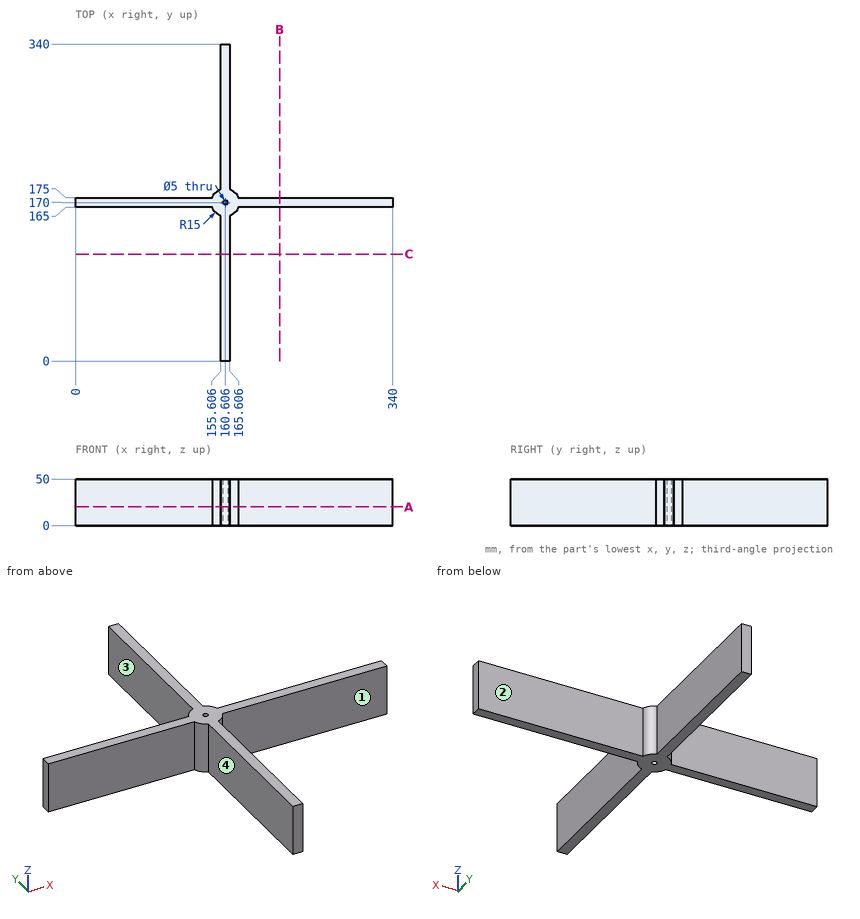
Verification items for this drawing (mm, ordinates from the low corner). A direction names the side the tool comes from. Give positions to 0.01 mm unless a question says otherwise; leave off trailing zeros. Loops run counter-clockwise (first coordinate to the right, second up) from the corner with the lowest first, then second, coordinate; pieces in that order, holes last. Notation, with made-up numbers: M 21.5,-31.5 L 62.5,-31.5 A22 ccw 62.5,-4.5 Z; hole C -11.5,31.25 d2. An arc over 180 degrees is marked long. Answer in a Markdown table with one row per item.
1) Thickness scan on line 1 (X direction, y = 170, z = 24); line 2 (X direction, y = 113, z = 5); line 3 (Y direction, x = 265.5, z = 2). Record the ranges inside material, lowest first.
Solutions:
| item | result |
|---|---|
| line 1 | x = 0 to 158.11, 163.11 to 340 |
| line 2 | x = 155.61 to 165.61 |
| line 3 | y = 165 to 175 |
2) Cross-section at A-A (z = 20). Enter the section's corners in (x, y), plus the area to 3 significant figures.
Solutions:
| item | result |
|---|---|
| outline | M 0,165 L 146.46,165 A15 ccw 155.61,155.86 L 155.61,0 L 165.61,0 L 165.61,155.86 A15 ccw 174.75,165 L 340,165 L 340,175 L 174.75,175 A15 ccw 165.61,184.14 L 165.61,340 L 155.61,340 L 155.61,184.14 A15 ccw 146.46,175 L 0,175 Z; hole C 160.61,170 d5 |
| area | 6,900 mm^2 |
3) Cross-section at C-C (y = 114.5). Enter the section's corners in (x, z).
Solutions:
| item | result |
|---|---|
| outline | M 155.61,0 L 165.61,0 L 165.61,50 L 155.61,50 Z |
4) Tool access check on the marked faces 1, 2, 3 and 4. Record the directions out of +Z, -Z, +X, -X, +Y, -Y that give a thin tool (end or side, any length) a straight path to the whole face; none if there is none.
Solutions:
| item | result |
|---|---|
| face 1 | +Z, -Z, +X, -Y |
| face 2 | +Z, -Z, +X, +Y |
| face 3 | +Z, -Z, -X, +Y |
| face 4 | +Z, -Z, -X, -Y |
5) Depth check by flat-ended pin: pin 1 (1 mm diameter, centred on x = 131, z = 22.5, fed in from -Y); pin 2 (4 mm diameter, centred on y = 45.5, z = 13, fed in from +X); pin 3 (1 mm diameter, centred on x = 235.5, z = 13.5, fed in from +Y). Enter the tip coordinate at first touch or a pass-through.
Solutions:
| item | result |
|---|---|
| pin 1 | stops at y = 165 |
| pin 2 | stops at x = 165.61 |
| pin 3 | stops at y = 175 |
6) Cross-section at B-B (x = 219). Enter the section's corners in (y, z), plus the area to 3 significant figures.
Solutions:
| item | result |
|---|---|
| outline | M 165,0 L 175,0 L 175,50 L 165,50 Z |
| area | 500 mm^2 |
